The drawing under review shows one solid part. Ordinate dimensions are in mm from its lowest x, y, z. Coordinates: 2 decimals unless noted, no trailing zeros. Write each loop counter-clockwise with the first axis right and the second up, starting at its lowest first coordinate (ties: lowest second). Pieces come first, ordered by that corner, then holes. Notation, with made-up numbers: (-2.75, 57.25) -> (29.25, 57.25) arc R14 ccw to (29.25, 74.25) -> close; hole circle Ø11 at (-4, 80.25). An arc over 180 degrees is marked (long way). One line per item, written item: value. Start each with the question number.
1) Mouldability with a two-part tool opening along Z and no side actions: class the marked faces 1 and 2 as released by +Z, released by -Z, zero draft, split by the parting line, or undercut.
2) For probe 1 along Z at (x, y) = (14.25, 3.75); probe 2 along X at (y, z) = (0.5, 19); probe 3 along X at (y, z) = (5.25, 5.5) (1 decimal), list the stretches that pass through material, from the lowest coordinate up. Write a range as from..to.
3) Add section C-C (y = 3). State the section outline as (x, z) points.
4) For pin 1 Ø0.5 at (x, y) = (15, 0.5) entering from -Z; pin 2 Ø0.8 at (x, y) = (17, 0.5) entering from +Z; pin 3 Ø1 at (y, z) = (2.5, 21.5) entering from +X, all flat-tipped, find the tip position at first contact; note any pin that passes through.
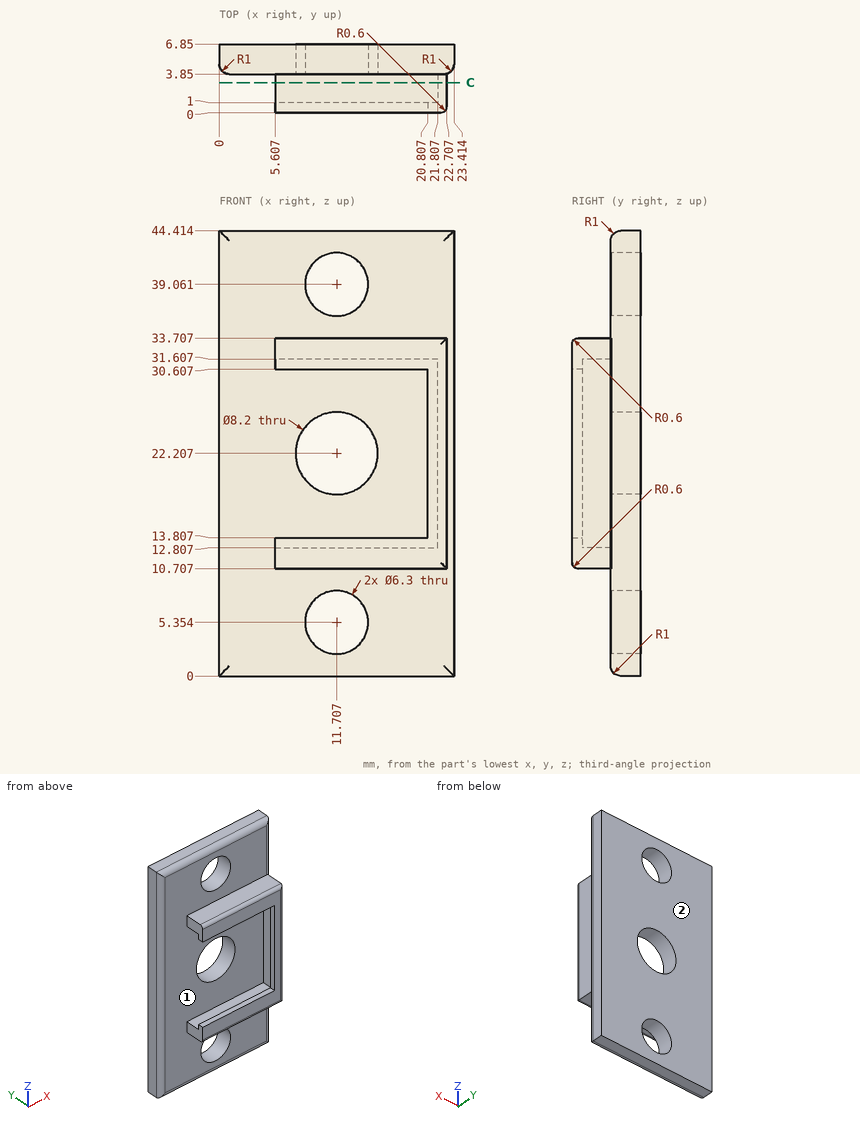
Numbers:
1. face 1: undercut
1. face 2: zero draft
2. probe 1: 10.71..12.81, 31.61..33.71
2. probe 2: 20.81..22.7
2. probe 3: 0..8.6, 14.9..23.4
3. outline: (5.61, 10.71) -> (22.71, 10.71) -> (22.71, 33.71) -> (5.61, 33.71) -> (5.61, 31.61) -> (21.81, 31.61) -> (21.81, 12.81) -> (5.61, 12.81) -> close
4. pin 1: z = 10.71
4. pin 2: z = 33.71
4. pin 3: x = 22.71
